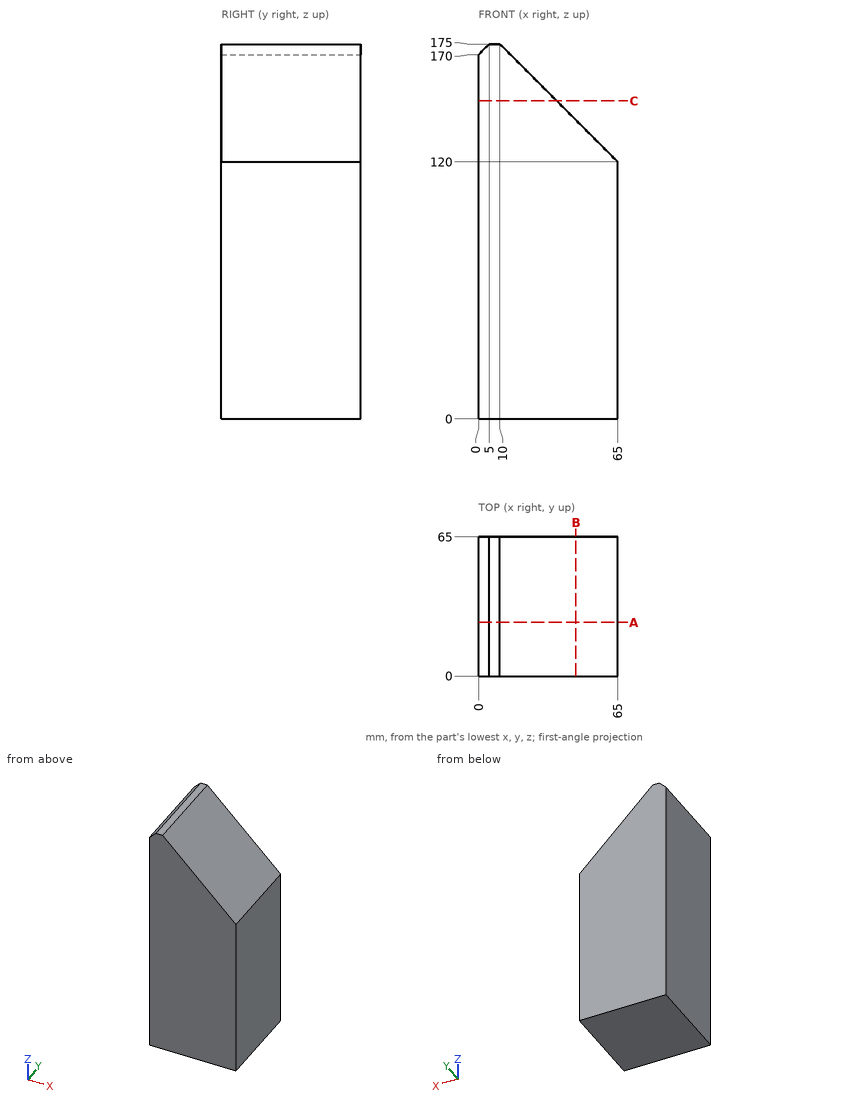
For this review, use the dimensioned drawing (mm, ordinates from the lowest corner) and the shaded views. Round coordinates to 2 decimals unless told otherwise and drop trailing zeros. Order: outer loops, then holes, each group sorted by start corner. A loop starts at its lowest first (then second) coordinate and runs counter-clockwise, first axis right, second up. Notation, with made-up numbers: (73, 25) -> (126, 25) arc R16 cw to (126, 39) -> close; hole circle Ø5 at (86, -24). An arc over 180 degrees is marked (long way). One line per item, written item: value. Start each with the question number.
Q1. Take a section at A-A (y = 25). Write out the cut boundary in (x, z), and give its area (3 significant figures).
Q2. Take a section at B-B (x = 45.5). Write out the cut boundary in (y, z), and give its area (3 significant figures).
Q3. Clearance check with flat-ended pins moving along their axes: pin 1 Ø4 at (x, y) = (40.5, 16) entering from +Z; pin 2 Ø1 at (x, y) = (50, 8.5) entering from +Z. State where each tip first meets the part, or that it passes through.
Q4. Take a section at C-C (z = 148.5). Write out the cut boundary in (x, y).
Q5. Wall thickness on line 1 (Z direction, x = 3.5, y = 8.5); line 2 (Z direction, x = 18.5, y = 41); line 3 (X direction, y = 42.5, z = 122): over which ranges is each line inside the solid? List them lowest first.
Reported:
1. outline: (0, 0) -> (65, 0) -> (65, 120) -> (10, 175) -> (5, 175) -> (0, 170) -> close
1. area: 9,850 mm2
2. outline: (0, 0) -> (65, 0) -> (65, 139.5) -> (0, 139.5) -> close
2. area: 9,070 mm2
3. pin 1: stops at z = 146.5
3. pin 2: stops at z = 135.5
4. outline: (0, 0) -> (36.5, 0) -> (36.5, 65) -> (0, 65) -> close
5. line 1: z = 0 to 173.5
5. line 2: z = 0 to 166.5
5. line 3: x = 0 to 63
